Verification items for the finished model (mm, model axes). A direction names the side the tool comes from. Round coordinates to 2 decimals unless told otherwise and drop trailing zeros. Write each loop counter-clockwise with the first axis right and the second up, starting at its lowest first coordinate (ties: lowest second). Pieces come first, ordered by that corner, then holes.
from build123d import *

# Parameters (mm, degrees)
SKETCH2_W           = 50
SKETCH2_H           = 50
BOSS_EXTRUDE1_DEPTH = 10
SKETCH3_W           = 7.5
SKETCH3_H           = 25
BOSS_EXTRUDE2_DEPTH = 35
SKETCH4_R           = 3.75
CUT_EXTRUDE1_DEPTH  = 50


with BuildPart() as part:
    # Sketch2 → Boss-Extrude1 (new body)
    with BuildSketch(Plane(origin=(0, 0, 0), x_dir=(1, 0, 0), z_dir=(0, 1, 0))):
        with Locations((25, 25)):
            Rectangle(SKETCH2_W, SKETCH2_H)
    extrude(amount=BOSS_EXTRUDE1_DEPTH)

    # Sketch3 → Boss-Extrude2 (add)
    with BuildSketch(Plane(origin=(0, 10, 0), x_dir=(1, 0, 0), z_dir=(0, 1, 0))):
        with Locations((3.75, 25)):
            Rectangle(SKETCH3_W, SKETCH3_H)
        with Locations((46.25, 25)):
            Rectangle(SKETCH3_W, SKETCH3_H)
    extrude(amount=BOSS_EXTRUDE2_DEPTH)

    # Sketch4 → Cut-Extrude1 (cut)
    with BuildSketch(Plane(origin=(50, 0, 0), x_dir=(0, 0, -1), z_dir=(1, 0, 0))):
        with Locations((25, 37.5)):
            Circle(SKETCH4_R)
    extrude(amount=-CUT_EXTRUDE1_DEPTH, mode=Mode.SUBTRACT)


solid = part.part
Q1. Sectioned sample at C-C (y = 30.5). Enter the section's corners in (x, z), plus the area to 3 significant figures.
Recorded:
outline: (0, -37.5) - (7.5, -37.5) - (7.5, -12.5) - (0, -12.5) - close; (42.5, -37.5) - (50, -37.5) - (50, -12.5) - (42.5, -12.5) - close
area: 375 mm2
Q2. Sectioned sample at A-A (z = -25). Enter the section's corners in (x, y), plus the area to 4 significant figures.
Recorded:
outline: (0, 0) - (50, 0) - (50, 33.75) - (42.5, 33.75) - (42.5, 10) - (7.5, 10) - (7.5, 33.75) - (0, 33.75) - close; (0, 41.25) - (7.5, 41.25) - (7.5, 45) - (0, 45) - close; (42.5, 41.25) - (50, 41.25) - (50, 45) - (42.5, 45) - close
area: 912.5 mm2
Q3. Sectioned sample at B-B (y = 37.5). Enter the section's corners in (x, z), plus the area to 4 significant figures.
Recorded:
outline: (0, -37.5) - (7.5, -37.5) - (7.5, -28.75) - (0, -28.75) - close; (0, -21.25) - (7.5, -21.25) - (7.5, -12.5) - (0, -12.5) - close; (42.5, -37.5) - (50, -37.5) - (50, -28.75) - (42.5, -28.75) - close; (42.5, -21.25) - (50, -21.25) - (50, -12.5) - (42.5, -12.5) - close
area: 262.5 mm2
Q4. Material ranges on line 1 along Y through (x, z) = (3, -25); line 2 along X through (y, z) = (32, -36); line 3 along Y through (x, z) = (14.5, -19.5), recorded low to high.
Recorded:
line 1: y = 0 to 33.75, 41.25 to 45
line 2: x = 0 to 7.5, 42.5 to 50
line 3: y = 0 to 10
Q5. Release check for a two-part mould opening along Z. For faces 1 (the cylindrical face through (3.803, 34.173, -26.73)), 2 (the flat face through (25, 5, -50)), 3 (the cylindrical face through (46.302, 34.173, -26.73)), 4 (the flat face through (0, 17, -25)) record: released by +Z, released by -Z, zero draft, split by the parting line, or undercut.
Recorded:
face 1: undercut
face 2: released by -Z
face 3: undercut
face 4: zero draft
Q6. Tool access check on faces 5 (the flat face through (46, 27, -12.5)), 6 (the flat face through (42.5, 27, -25)), 7 (the flat face through (25, 0, -25)), 8 (the flat face through (46, 27, -37.5)), 9 (the flat face through (50, 17, -25)). Record the directions out of +Z, -Z, +X, -X, +Y, -Y that give a thin tool (end or side, any length) a straight path to the whole face; none if there is none.
Recorded:
face 5: +Z, +X, -X, +Y
face 6: +Z, -Z, +Y
face 7: +Z, -Z, +X, -X, -Y
face 8: -Z, +X, -X, +Y
face 9: +Z, -Z, +X, +Y, -Y
Q7. Sectioned sample at D-D (z = -15.5). Enter the section's corners in (x, y), plus the area to 4 significant figures.
Recorded:
outline: (0, 0) - (50, 0) - (50, 45) - (42.5, 45) - (42.5, 10) - (7.5, 10) - (7.5, 45) - (0, 45) - close
area: 1,025 mm2
Q8. Depth check by flat-ended pin: P1, Ø1.5, axis at x = 16.5, z = -20.5, coming from the -Y side; P2, Ø12, axis at x = 7, y = 30, coming from the +Z side; P3, Ø2, axis at x = 2, y = 35.5, coming from the -Z side; P4, Ø1.5, axis at x = 5.5, z = -8.5, coming from the +Y side. Enter the tip coordinate at first touch or a pass-through.
Recorded:
P1: stops at y = 0
P2: stops at z = -12.5
P3: stops at z = -37.5
P4: stops at y = 10
